from build123d import *

# Parameters (mm, degrees)
BOSS_EXTRUDE1_DEPTH = 1
BOSS_EXTRUDE2_DEPTH = 20
CUT_EXTRUDE1_DEPTH  = 2
SKETCH3_R           = 1.175
CUT_EXTRUDE2_DEPTH  = 20
MOVE_FACE1_BY       = 0.2
MOVE_FACE1_2_BY     = 0.2
MOVE_FACE1_3_BY     = 0.2
MOVE_FACE1_4_BY     = 0.2
MOVE_FACE1_5_BY     = 0.2
MOVE_START          = 1
MOVE_FACE2_DEPTH    = 19


# Read off the part's stored shape, not the designer's step: Move Face2
with BuildPart() as part:
    # Sketch1 → Boss-Extrude1 (new body)
    with BuildSketch(Plane(origin=(0, 0, 0), x_dir=(1, 0, 0), z_dir=(0, 1, 0))):
        with BuildLine():
            Line((-11.433858941, 48.348949441), (-21.758858941, 48.348949441))
            Line((-21.758858941, 48.348949441), (-30.758858941, 48.348949441))
            Line((-30.758858941, 48.348949441), (-41.083858941, 48.348949441))
            ThreePointArc((-41.083858941, 48.348949441), (-42.498072504, 47.763163004), (-43.083858941, 46.348949441))
            Line((-43.083858941, 46.348949441), (-46.733732675, 43.323823175))
            ThreePointArc((-46.733732675, 43.323823175), (-47.758858941, 40.848949441), (-46.733732675, 38.374075707))
            Line((-46.733732675, 38.374075707), (-43.083858941, 35.348949441))
            ThreePointArc((-43.083858941, 35.348949441), (-42.498072504, 33.934735879), (-41.083858941, 33.348949441))
            Line((-41.083858941, 33.348949441), (-11.433858941, 33.348949441))
            ThreePointArc((-11.433858941, 33.348949441), (-10.019645379, 33.934735879), (-9.433858941, 35.348949441))
            Line((-9.433858941, 35.348949441), (-5.783985207, 38.374075707))
            ThreePointArc((-5.783985207, 38.374075707), (-4.758858941, 40.848949441), (-5.783985207, 43.323823175))
            Line((-5.783985207, 43.323823175), (-9.433858941, 46.348949441))
            ThreePointArc((-9.433858941, 46.348949441), (-10.019645379, 47.763163004), (-11.433858941, 48.348949441))
        make_face()
    extrude(amount=BOSS_EXTRUDE1_DEPTH)

    # Sketch1<3> → Boss-Extrude2 (add)
    with BuildSketch(Plane(origin=(0, 0, 0), x_dir=(1, 0, 0), z_dir=(0, 1, 0))):
        with BuildLine():
            Line((-21.758858941, 50.348949441), (-30.758858941, 50.348949441))
            Line((-30.758858941, 50.348949441), (-41.083858941, 50.348949441))
            ThreePointArc((-41.083858941, 50.348949441), (-43.509516051, 49.529544917), (-44.941375957, 47.407043233))
            Line((-44.941375957, 47.407043233), (-48.073804253, 44.810791471))
            ThreePointArc((-48.073804253, 44.810791471), (-49.758858941, 40.848949441), (-48.073804253, 36.887107411))
            Line((-48.073804253, 36.887107411), (-44.941375957, 34.290855649))
            ThreePointArc((-44.941375957, 34.290855649), (-43.509516051, 32.168353965), (-41.083858941, 31.348949441))
            Line((-41.083858941, 31.348949441), (-11.433858941, 31.348949441))
            ThreePointArc((-11.433858941, 31.348949441), (-9.008201831, 32.168353965), (-7.576341925, 34.290855649))
            Line((-7.576341925, 34.290855649), (-4.443913629, 36.887107411))
            ThreePointArc((-4.443913629, 36.887107411), (-2.758858941, 40.848949441), (-4.443913629, 44.810791471))
            Line((-4.443913629, 44.810791471), (-7.576341925, 47.407043233))
            ThreePointArc((-7.576341925, 47.407043233), (-9.008201831, 49.529544917), (-11.433858941, 50.348949441))
            Line((-11.433858941, 50.348949441), (-21.758858941, 50.348949441))
        make_face()
        with BuildLine():
            Line((-11.433858941, 48.348949441), (-21.758858941, 48.348949441))
            Line((-21.758858941, 48.348949441), (-30.758858941, 48.348949441))
            Line((-30.758858941, 48.348949441), (-41.083858941, 48.348949441))
            ThreePointArc((-41.083858941, 48.348949441), (-42.498072504, 47.763163004), (-43.083858941, 46.348949441))
            Line((-43.083858941, 46.348949441), (-46.733732675, 43.323823175))
            ThreePointArc((-46.733732675, 43.323823175), (-47.758858941, 40.848949441), (-46.733732675, 38.374075707))
            Line((-46.733732675, 38.374075707), (-43.083858941, 35.348949441))
            ThreePointArc((-43.083858941, 35.348949441), (-42.498072504, 33.934735879), (-41.083858941, 33.348949441))
            Line((-41.083858941, 33.348949441), (-11.433858941, 33.348949441))
            ThreePointArc((-11.433858941, 33.348949441), (-10.019645379, 33.934735879), (-9.433858941, 35.348949441))
            Line((-9.433858941, 35.348949441), (-5.783985207, 38.374075707))
            ThreePointArc((-5.783985207, 38.374075707), (-4.758858941, 40.848949441), (-5.783985207, 43.323823175))
            Line((-5.783985207, 43.323823175), (-9.433858941, 46.348949441))
            ThreePointArc((-9.433858941, 46.348949441), (-10.019645379, 47.763163004), (-11.433858941, 48.348949441))
        make_face(mode=Mode.SUBTRACT)
    extrude(amount=BOSS_EXTRUDE2_DEPTH)

    # Sketch2 → Cut-Extrude1 (cut)
    with BuildSketch(Plane.XY.offset(-50.348949441)):
        Polygon((-21.758858941, 1), (-21.758858941, 6), (-30.758858941, 6), (-30.758858941, 1), (-30.758858941, 0), (-21.758858941, 0), align=None)
    extrude(amount=CUT_EXTRUDE1_DEPTH, mode=Mode.SUBTRACT)

    # Sketch3 → Cut-Extrude2 (cut)
    with BuildSketch(Plane(origin=(0, 1, 0), x_dir=(1, 0, 0), z_dir=(0, 1, 0))):
        with Locations(Location((-8.258858941, 40.848949441, 0), (0, 0, 270))):
            Circle(SKETCH3_R)
        with Locations(Location((-44.258858941, 40.848949441, 0), (0, 0, 270))):
            Circle(SKETCH3_R)
    extrude(amount=-CUT_EXTRUDE2_DEPTH, mode=Mode.SUBTRACT)

    # Move Face1: a face moved inward by 0.2
    extrude(part.faces().sort_by_distance((-26.258858941, 6, -49.348949441))[0], amount=MOVE_FACE1_BY, dir=(0, 1, 0), mode=Mode.SUBTRACT)

    # Move Face1 2: a face moved inward by 0.2
    extrude(part.faces().sort_by_distance((-30.758858941, 3, -49.348949441))[0], amount=MOVE_FACE1_2_BY, dir=(-1, 0, 0), mode=Mode.SUBTRACT)

    # Move Face1 3: a face moved inward by 0.2
    extrude(part.faces().sort_by_distance((-21.758858941, 3, -49.348949441))[0], amount=MOVE_FACE1_3_BY, dir=(1, 0, 0), mode=Mode.SUBTRACT)

    # Move Face1 4: a curved face moved inward by 0.2
    add(Solid.thicken(part.faces().sort_by_distance((-44.258858941, 0.5, -42.023949441))[0], -MOVE_FACE1_4_BY), mode=Mode.SUBTRACT)

    # Move Face1 5: a curved face moved inward by 0.2
    add(Solid.thicken(part.faces().sort_by_distance((-8.258858941, 0.5, -42.023949441))[0], -MOVE_FACE1_5_BY), mode=Mode.SUBTRACT)

    # Move Face2 outline → Move Face2 (cut)
    with BuildSketch(Plane(origin=(0, 0, 0), x_dir=(1, 0, 0), z_dir=(0, 1, 0)).offset(MOVE_START)):
        with BuildLine():
            ThreePointArc((-41.083858941, 48.848949441), (-42.762782817, 48.201303246), (-43.571827765, 46.593921137))
            Line((-43.571827765, 46.593921137), (-47.070175615, 43.694384128))
            ThreePointArc((-47.070175615, 43.694384128), (-48.258858941, 40.848949441), (-47.070175615, 38.003514754))
            Line((-47.070175615, 38.003514754), (-43.571827765, 35.103977746))
            ThreePointArc((-43.571827765, 35.103977746), (-42.762782817, 33.496595636), (-41.083858941, 32.848949441))
            Line((-41.083858941, 32.848949441), (-11.433858941, 32.848949441))
            ThreePointArc((-11.433858941, 32.848949441), (-9.754935065, 33.496595636), (-8.945890117, 35.103977746))
            Line((-8.945890117, 35.103977746), (-5.447542267, 38.003514754))
            ThreePointArc((-5.447542267, 38.003514754), (-4.258858941, 40.848949441), (-5.447542267, 43.694384128))
            Line((-5.447542267, 43.694384128), (-8.945890117, 46.593921137))
            ThreePointArc((-8.945890117, 46.593921137), (-9.754935065, 48.201303246), (-11.433858941, 48.848949441))
            Line((-11.433858941, 48.848949441), (-41.083858941, 48.848949441))
        make_face()
        with BuildLine():
            Line((-41.083858941, 48.348949441), (-11.433858941, 48.348949441))
            ThreePointArc((-11.433858941, 48.348949441), (-10.019645379, 47.763163004), (-9.433858941, 46.348949441))
            Line((-9.433858941, 46.348949441), (-5.783985207, 43.323823175))
            ThreePointArc((-5.783985207, 43.323823175), (-4.758858941, 40.848949441), (-5.783985207, 38.374075707))
            Line((-5.783985207, 38.374075707), (-9.433858941, 35.348949441))
            ThreePointArc((-9.433858941, 35.348949441), (-10.019645379, 33.934735879), (-11.433858941, 33.348949441))
            Line((-11.433858941, 33.348949441), (-41.083858941, 33.348949441))
            ThreePointArc((-41.083858941, 33.348949441), (-42.498072504, 33.934735879), (-43.083858941, 35.348949441))
            Line((-43.083858941, 35.348949441), (-46.733732675, 38.374075707))
            ThreePointArc((-46.733732675, 38.374075707), (-47.758858941, 40.848949441), (-46.733732675, 43.323823175))
            Line((-46.733732675, 43.323823175), (-43.083858941, 46.348949441))
            ThreePointArc((-43.083858941, 46.348949441), (-42.498072504, 47.763163004), (-41.083858941, 48.348949441))
        make_face(mode=Mode.SUBTRACT)
    extrude(amount=MOVE_FACE2_DEPTH, mode=Mode.SUBTRACT)


solid = part.part
CAD build for the part. Positions are in the model's coordinates, mm. A direction names the side the tool comes from. Round coordinates to 2 decimals unless told otherwise and drop trailing zeros. Write each loop counter-clockwise with the first axis right and the second up, starting at its lowest first coordinate (ties: lowest second). Pieces come first, ordered by that corner, then holes.
(1) Slice it at D-D, the plane y = 4. Write the cut outline in (x, z), and give its area (3 significant figures).
(2) Slice it at B-B, the plane y = 14.5. Write the cut outline in (x, z).
(3) Mould opens along X. For faces 4 (the face through (-45.3, 10.37, -45.16)), 5 (the face through (-27, 0, -41)), 6 (the face through (-8.98, 9.86, -49.51)), 7 (the face through (-21.559, 3, -50)) say: pulls with the +X half, pulls with the -X half, needs draft (parallel to the pull), parting line crosses it, or undercut.
(4) Slice it at C-C, the plane z = -40. Write the cut outline in (x, y), and give its area (4 significant figures).
(5) Drop flat-ended pins along their axis: P1, Ø0.8, axis at x = -26.5, z = -50, coming from the -Y side; P2, Ø1.6, axis at y = 4.5, z = -49, coming from the -X side; P3, Ø5, axis at x = -23, z = -42.5, coming from the +Y side; P4, Ø1.6, axis at x = -8.26, z = -40.85, coming from the -Y side. Give the stop position or say it passes through.
(6) 3-axis set-ups, long thin cutter, end or side, ignore diameter. For faces 1 (the face through (-43.48, 9.86, -49.55)), 2 (the face through (-45.345, 10.367, -36.574)), 3 (the face through (-26, 6.2, -50)): which of +Z, -Z, +X, -X, +Y, -Y reach the whole face in a straight line?
(7) Slice it at A-A, the plane x = -28. Write the cut outline in (y, z).
(8) Probe line 1 along Z through (x, y) = (-36, 13); line 2 along Y through (x, z) = (-11, -40.75); line 3 along X through (y, z) = (4.5, -39). List the from-to ranges inside material, lowest first.
From the geometry:
1. outline: (-48.07, -44.81) - (-44.94, -47.41) arc R4 ccw to (-41.08, -50.35) - (-30.96, -50.35) - (-30.96, -48.85) - (-41.08, -48.85) arc R2.5 cw to (-43.57, -46.59) - (-47.07, -43.69) arc R4 cw to (-47.07, -38) - (-43.57, -35.1) arc R2.5 cw to (-41.08, -32.85) - (-11.43, -32.85) arc R2.5 cw to (-8.95, -35.1) - (-5.45, -38) arc R4 cw to (-5.45, -43.69) - (-8.95, -46.59) arc R2.5 cw to (-11.43, -48.85) - (-21.56, -48.85) - (-21.56, -50.35) - (-11.43, -50.35) arc R4 ccw to (-7.58, -47.41) - (-4.44, -44.81) arc R5.5 ccw to (-4.44, -36.89) - (-7.58, -34.29) arc R4 ccw to (-11.43, -31.35) - (-41.08, -31.35) arc R4 ccw to (-44.94, -34.29) - (-48.07, -36.89) arc R5.5 ccw to start
1. area: 150 mm2
2. outline: (-48.07, -44.81) - (-44.94, -47.41) arc R4 ccw to (-41.08, -50.35) - (-11.43, -50.35) arc R4 ccw to (-7.58, -47.41) - (-4.44, -44.81) arc R5.5 ccw to (-4.44, -36.89) - (-7.58, -34.29) arc R4 ccw to (-11.43, -31.35) - (-41.08, -31.35) arc R4 ccw to (-44.94, -34.29) - (-48.07, -36.89) arc R5.5 ccw to start; hole (-47.07, -43.69) - (-43.57, -46.59) arc R2.5 ccw to (-41.08, -48.85) - (-11.43, -48.85) arc R2.5 ccw to (-8.95, -46.59) - (-5.45, -43.69) arc R4 ccw to (-5.45, -38) - (-8.95, -35.1) arc R2.5 ccw to (-11.43, -32.85) - (-41.08, -32.85) arc R2.5 ccw to (-43.57, -35.1) - (-47.07, -38) arc R4 ccw to start
3. face 4: undercut
3. face 5: needs draft
3. face 6: pulls with the +X half
3. face 7: undercut
4. outline: (-49.69, 0) - (-45.34, 0) - (-45.34, 1) - (-48.17, 1) - (-48.17, 20) - (-49.69, 20) - close; (-43.18, 0) - (-9.34, 0) - (-9.34, 1) - (-43.18, 1) - close; (-7.18, 0) - (-2.82, 0) - (-2.82, 20) - (-4.35, 20) - (-4.35, 1) - (-7.18, 1) - close
4. area: 100.5 mm2
5. P1: stops at y = 6.2
5. P2: stops at x = -44.63
5. P3: stops at y = 1
5. P4: passes through
6. face 1: -Z, -X, +Y, -Y
6. face 2: +Y
6. face 3: -Z, -Y
7. outline: (0, -48.35) - (1, -48.35) - (1, -32.85) - (20, -32.85) - (20, -31.35) - (0, -31.35) - close; (6.2, -50.35) - (20, -50.35) - (20, -48.85) - (6.2, -48.85) - close
8. line 1: z = -50.35 to -48.85, -32.85 to -31.35
8. line 2: y = 0 to 1
8. line 3: x = -49.44 to -47.81, -4.71 to -3.08
